Input: dimensioned drawing with shaded views. Units: mm. Origin: part minimum x, y, z. A direction names the side the tool comes from. Coordinates: 2 decimals unless noted, no trailing zeros. Write each loop counter-clockwise with the first axis right and the second up, starting at its lowest first coordinate (ties: lowest second). Pieces come first, ordered by that corner, then holes. Notation, with made-up numbers: M -14,52.25 L 36,52.25 A22 ccw 36,64.25 Z; hole C 58,76.5 d6. An arc over 180 degrees is marked long. Use one line per item in the form item = value.
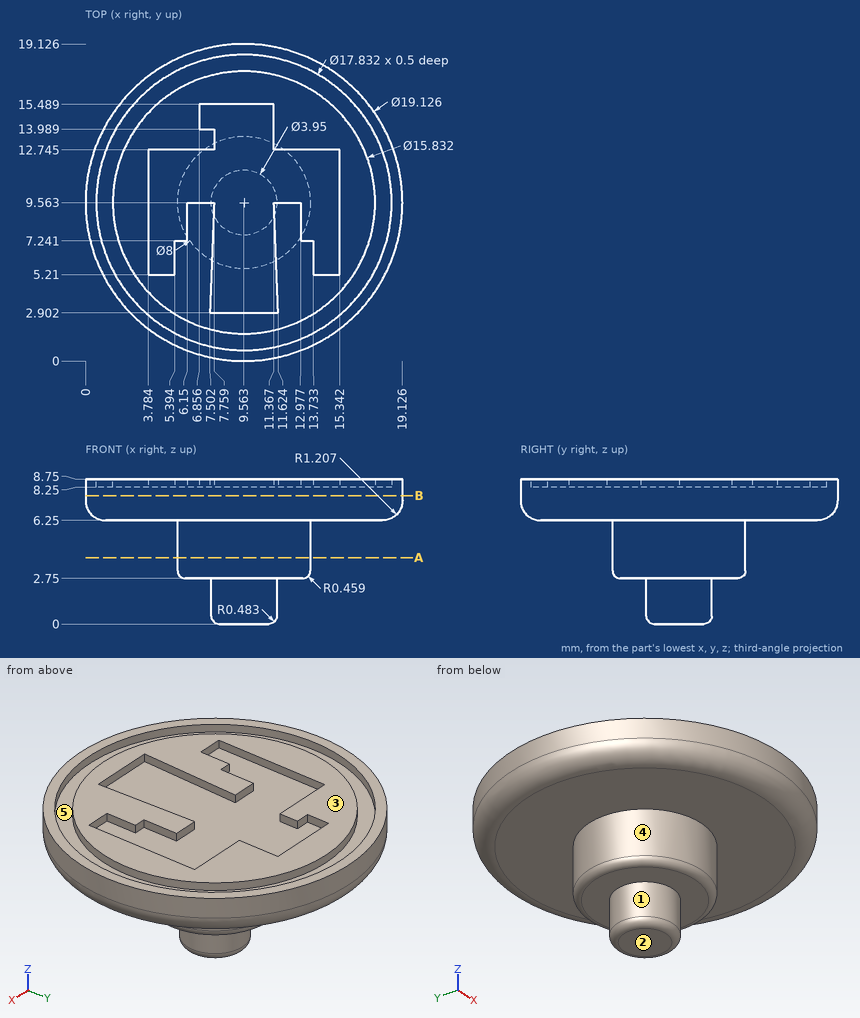
(1) Section query B-B on z = 7.75. Return the cut outline in (x, y), plus the area to 3 significant figures.
Computed:
outline = C 9.56,9.56 d19.13
area = 287 mm^2
(2) Section query A-A on z = 4. Return the cut outline in (x, y).
Computed:
outline = C 9.56,9.56 d8
(3) First-contact query: pin 1 Ø2 at (y, z) = (5, 2) entering from -X; pin 2 Ø0.6 at (y, z) = (13.5, 8.5) entering from -X; pin 3 Ø0.6 at (y, z) = (15, 8.5) entering from +X; pin 4 Ø0.6 at (x, z) = (13.5, 8.5) entering from +Y. Flat tips, straight axial feed; report the tip coordinate or a pass-through.
Computed:
pin_1 = through
pin_2 = 0.72
pin_3 = 17.63
pin_4 = 18.41
(4) Set-up query: the marked faces 1 and 2. Return all of +Z, -Z, +X, -X, +Y, -Y with unobstructed straight access to the full face (end or side cutting, diameter ignored); none if empty.
Computed:
face_1 = -Z
face_2 = -Z, +X, -X, +Y, -Y
(5) Line query: probe 1 along Z at (x, y) = (14.5, 10.5); probe 2 along Z at (x, y) = (8.5, 2.75); probe 3 along Y at (x, z) = (8.75, 0.5) (1 decimal). Output: solid intervals per line, ascending.
Computed:
probe_1 = 6.25 to 8.25
probe_2 = 6.25 to 8.75
probe_3 = 7.8 to 11.4
(6) Pull-direction query (Y, two-part tool) for the marked faces 3, 4 and 5; classes: pulls with the +Y half, pulls with the -Y half, needs draft (parallel to the pull), parting line crosses it, or undercut.
Computed:
face_3 = needs draft
face_4 = parting line crosses it
face_5 = undercut
